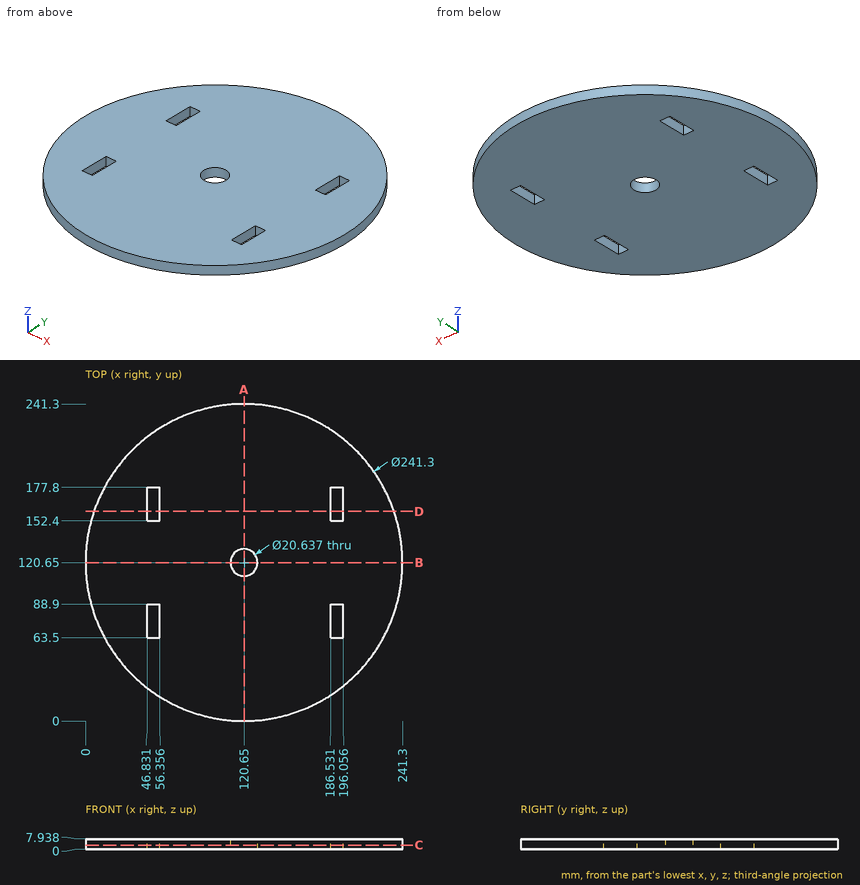
Here's the drawing with two shaded views (mm, measured from the low corner). I have some questions. Give positions to 0.01 mm unless a question says otherwise; leave off trailing zeros. Write each loop counter-clockwise with the first axis right and the second up, starting at its lowest first coordinate (ties: lowest second). Pieces come first, ordered by that corner, then holes. Notation, with made-up numbers: (10, 2) - (33, 2) arc R18 cw to (33, 25) - close; hole circle Ø10 at (30.5, 65.5). An arc over 180 degrees is marked (long way). One line per item, written item: value. Start each with the question number.
Item 1: Imagine slicing it at C-C, the plane z = 3.25. List the corners of the cut face in (x, y) for me.
Item 2: Imagine slicing it at D-D, the plane y = 159.5. List the corners of the cut face in (x, z) for me.
Item 3: I'm going to push flat-ended pins straight in: pin 1 (1.5 mm diameter, centred on x = 82, z = 3, fed in from +Y); pin 2 (4 mm diameter, centred on x = 52.5, z = 4, fed in from -Y); pin 3 (1.5 mm diameter, centred on y = 87.5, z = 3, fed in from +X); pin 4 (18.5 mm diameter, centred on x = 120.65, y = 120.65, fed in from +Z). Where does each tip first touch, or does it pass through?
Item 4: Imagine slicing it at A-A, the plane x = 120.65. List the corners of the cut face in (y, z) for me, and give its area (3 significant figures).
Item 5: Please list where these lines run through material, in increasing order: line 1 (Y direction, x = 120.65, z = 3.5); line 2 (Y direction, x = 194.5, z = 4.25) (1 decimal); line 3 (X direction, y = 170, z = 0.5) (1 decimal). Write a range as from..to.
Geometry says:
1. outline: circle Ø241.3 at (120.65, 120.65); hole (46.83, 63.5) - (56.36, 63.5) - (56.36, 88.9) - (46.83, 88.9) - close; hole (46.83, 152.4) - (56.36, 152.4) - (56.36, 177.8) - (46.83, 177.8) - close; hole circle Ø20.64 at (120.65, 120.65); hole (186.53, 63.5) - (196.06, 63.5) - (196.06, 88.9) - (186.53, 88.9) - close; hole (186.53, 152.4) - (196.06, 152.4) - (196.06, 177.8) - (186.53, 177.8) - close
2. outline: (6.43, 0) - (46.83, 0) - (46.83, 7.94) - (6.43, 7.94) - close; (56.36, 0) - (186.53, 0) - (186.53, 7.94) - (56.36, 7.94) - close; (196.06, 0) - (234.87, 0) - (234.87, 7.94) - (196.06, 7.94) - close
3. pin 1: y = 235.19
3. pin 2: y = 19.75
3. pin 3: x = 236.87
3. pin 4: through
4. outline: (0, 0) - (110.33, 0) - (110.33, 7.94) - (0, 7.94) - close; (130.97, 0) - (241.3, 0) - (241.3, 7.94) - (130.97, 7.94) - close
4. area: 1,750 mm^2
5. line 1: 0..110.33, 130.97..241.3
5. line 2: 25.2..63.5, 88.9..152.4, 177.8..216.1
5. line 3: 10.6..46.8, 56.4..186.5, 196.1..230.7
